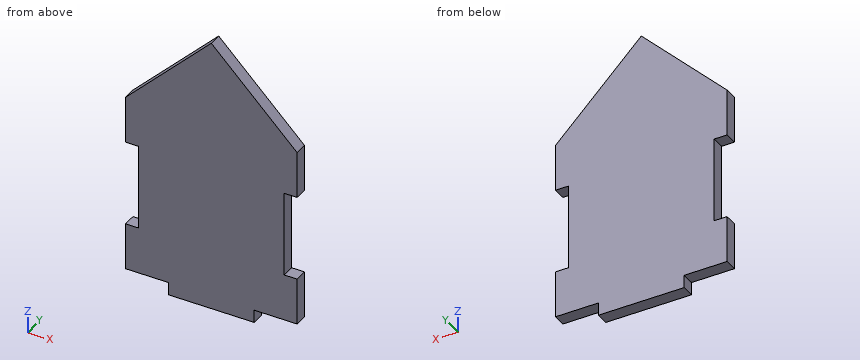
from build123d import *

# Parameters (mm, degrees)
F0_W     = 20
F0_H     = 40
F0_H_2   = 3
F1_DEPTH = 3


# Not quite as in the source:
# - a feature names something its author has since deleted; it is built from what else it names


with BuildPart() as f1:
    # F0 (on Front) → F1 (new body)
    with BuildSketch(Plane.XZ):
        Polygon((10, -21), (20, -21), (20, -10), (17, -10), (17, 10), (20, 10), (20, 21), (0, 41), (-20, 21), (-20, 10), (-17, 10), (-17, -10), (-20, -10), (-20, -21), (-10, -21), (-10, 19), (10, 19), align=None)
        with Locations((0, -1)):
            Rectangle(F0_W, F0_H)
        with Locations((0, -22.5)):
            Rectangle(F0_W, F0_H_2)
    extrude(amount=-F1_DEPTH)


solid = f1.part
The listing builds one solid part. Answer for the finished solid, in the listing's coordinates (mm). Round coordinates to 2 decimals unless told otherwise and drop trailing zeros. Write each loop counter-clockwise with the first axis right and the second up, starting at its lowest first coordinate (ties: lowest second). Pieces come first, ordered by that corner, then holes. Notation, with made-up numbers: (-13.5, 54) - (21.5, 54) arc R19 cw to (21.5, 88) - close; hole circle Ø8 at (23, -23). An arc over 180 degrees is marked (long way). Use a Markdown table: item, result. Add a question column.
1. The part is cut by section B-B (x = -6.5). Write down the section's boundary in (y, z).
2. The part is cut by section A-A (y = 0.8). Write down the section's boundary in (x, z).
3. Consider line 1 (X direction, y = 1.2, z = -1); line 2 (Z direction, x = 12, y = 2.1); line 3 (Z direction, x = 3, y = 2.4). Determine where each line is inside the solid, lowest interval first.
4. The part is cut by section C-C (z = 22). Write down the section's boundary in (x, y).
5. Flat-ended cylindrical pins translate along their axes: P1, Ø1.5, axis at x = -18.5, y = 1, coming from the +Z side; P2, Ø1.5, axis at x = 19, y = 2, coming from the -Z side; P3, Ø1.5, axis at y = 1.5, z = -22, coming from the +X side. Find the tip coordinate at first contact, or state that the pin passes through.
Reported:
| question | item | result |
|---|---|---|
| 1 | outline | (0, -24) - (3, -24) - (3, 34.5) - (0, 34.5) - close |
| 2 | outline | (-20, -21) - (-10, -21) - (-10, -24) - (10, -24) - (10, -21) - (20, -21) - (20, -10) - (17, -10) - (17, 10) - (20, 10) - (20, 21) - (0, 41) - (-20, 21) - (-20, 10) - (-17, 10) - (-17, -10) - (-20, -10) - close |
| 3 | line 1 | -17 to 17 |
| 3 | line 2 | -21 to 29 |
| 3 | line 3 | -24 to 38 |
| 4 | outline | (-19, 0) - (19, 0) - (19, 3) - (-19, 3) - close |
| 5 | P1 | z = 23.25 |
| 5 | P2 | z = -21 |
| 5 | P3 | x = 10 |
